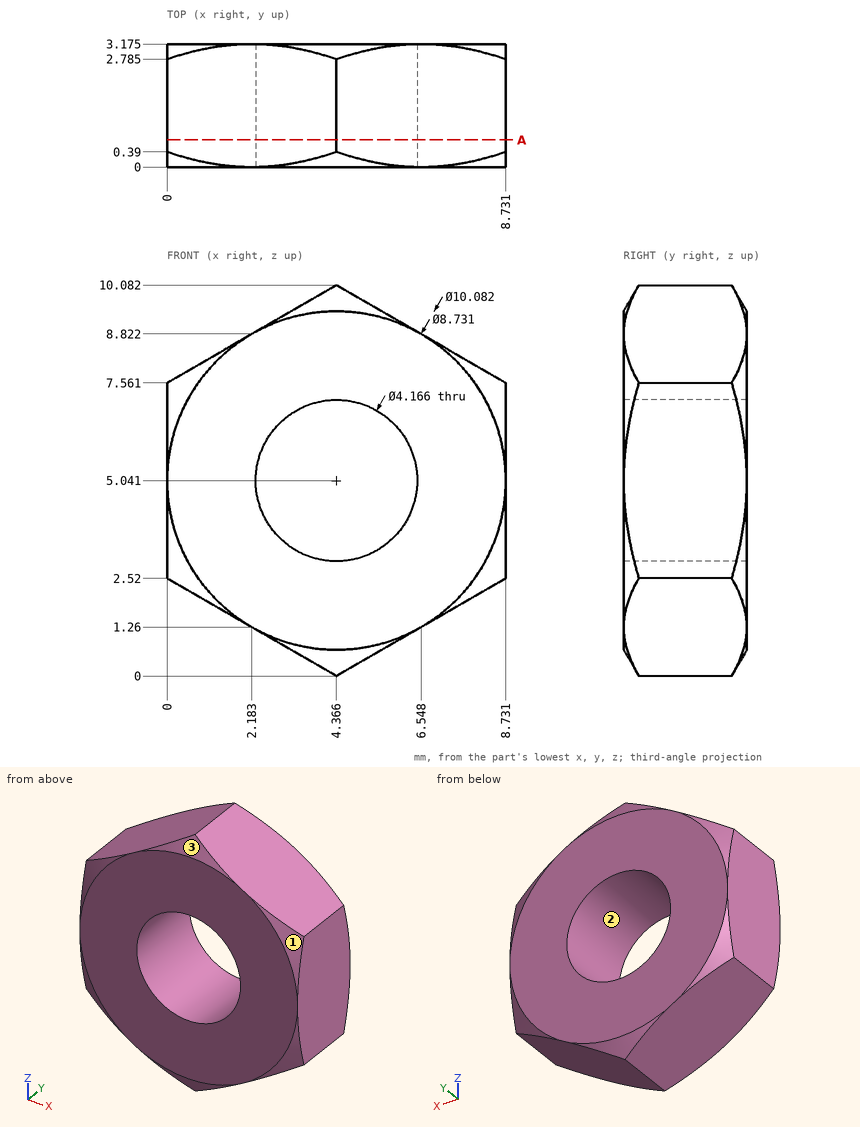
Input: dimensioned drawing with shaded views. Units: mm. Origin: part minimum x, y, z. Round coordinates to 2 decimals unless told otherwise and drop trailing zeros. Loops run counter-clockwise (first coordinate to the right, second up) from the corner with the lowest first, then second, coordinate; pieces in that order, holes last. Notation, with made-up numbers: M 28,-5.5 L 33,-5.5 A7 ccw 33,-1.5 Z; hole C 23,-5.5 d1. An arc over 180 degrees is marked long. Return JSON: item names as keys, results as strings. Group by question number.
1. Material intervals for line 1 along X through (y, z) = (2.05, 5); line 2 along Z through (x, y) = (5, 2.55) (1 decimal); line 3 along X through (y, z) = (2.15, 3.5) (1 decimal), sorted ascending. Write a range as from..to.
2. Pin query (flat end, axial travel): pin 1 (1.5 mm diameter, centred on y = 2.5, z = 8.5, fed in from +X) (1 decimal). Return the tip coordinate at first contact, or that it passes through.
3. Mould query, pull axis X, two halves, no side actions, for the marked faces 1, 2 and 3. Classes: released by +X, released by -X, zero draft, split by the parting line, or undercut.
4. Section query A-A on y = 0.7. Output: boundary loops of the cut face in (x, z) (1 decimal).
Checks:
{
 "1": {"line 1": "x = 0..2.28, 6.45..8.73", "line 2": "z = 0.4..3.1, 7..9.7", "line 3": "x = 0..3, 5.8..8.7"},
 "2": {"pin 1": "stops at x = 8.4"},
 "3": {"face 1": "released by +X", "face 2": "undercut", "face 3": "split by the parting line"},
 "4": {"outline": "M 0,2.5 L 4.4,0 L 8.7,2.5 L 8.7,7.6 L 4.4,10.1 L 0,7.6 Z; hole C 4.4,5 d4.2"}
}
